from build123d import *

# Parameters (mm, degrees)
SKETCH_1_W          = 145
SKETCH_1_H          = 163.96571483
F_145X120X4MM_DEPTH = 4
SKETCH_2_R          = 2.75
M3_90X70MM_DEPTH    = 162.686711765
FILLET_R5_R         = 5


with BuildPart() as part:
    # 草图1 → 承托板_145x120x4mm (new body)
    with BuildSketch(Plane(origin=(0, 0, 0), x_dir=(1, 0, 0), z_dir=(0, 1, 0))):
        with Locations((0, -62.482857415)):
            Rectangle(SKETCH_1_W, SKETCH_1_H)
    extrude(amount=F_145X120X4MM_DEPTH)

    # 草图2 → 四个M3连接孔_90x70mm (cut, through all)
    with BuildSketch(Plane(origin=(0, 4, 0), x_dir=(1, 0, 0), z_dir=(0, 1, 0))):
        with Locations(Location((-50, -8, 0), (0, 0, 270))):
            Circle(SKETCH_2_R)
        with Locations(Location((-50, -78, 0), (0, 0, 270))):
            Circle(SKETCH_2_R)
        with Locations(Location((50, -8, 0), (0, 0, 270))):
            Circle(SKETCH_2_R)
        with Locations(Location((50, -78, 0), (0, 0, 270))):
            Circle(SKETCH_2_R)
    extrude(amount=-M3_90X70MM_DEPTH, mode=Mode.SUBTRACT)

    # 四角圆角_R5
    fillet_r5_edges = [part.edges().sort_by_distance(p)[0] for p in [
        (-72.5, 2, -19.5),
        (72.5, 2, -19.5),
        (72.5, 2, 144.46571483),
        (-72.5, 2, 144.46571483),
    ]]
    fillet(fillet_r5_edges, radius=FILLET_R5_R)


solid = part.part
Geometry: final body of the model. Coordinates: model frame, mm. Coordinates: 2 decimals unless noted, no trailing zeros. Write each loop counter-clockwise with the first axis right and the second up, starting at its lowest first coordinate (ties: lowest second). Pieces come first, ordered by that corner, then holes. Notation, with made-up numbers: (27.5, 59) - (34.5, 59) arc R22 ccw to (34.5, 78) - close; hole circle Ø4 at (-25, 4). An arc over 180 degrees is marked (long way). Return JSON: item names as keys, results as strings.
Item 1: Pin query (flat end, axial travel): pin 1 Ø5 at (x, z) = (-50, 78) entering from +Y. Return the tip coordinate at first contact, or that it passes through.
Completed:
{"pin 1": "passes through"}
Item 2: Pull-direction query (X, two-part tool) for faces 1 (the face through (-71.074, 2.028, 142.962)), 2 (the face through (-48.141, 2.028, 75.973)), 3 (the face through (-47.273, 2.028, 7.642)), 4 (the face through (-1, 0, 61)); classes: +X half, -X half, draft (parallel to the pull), parting line (faces both ways), or undercut.
Completed:
{"face 1": "-X half", "face 2": "undercut", "face 3": "undercut", "face 4": "draft"}
Item 3: Section query B-B (z = 78). Output: boundary loops of the cut face in (x, y), and give its area (3 significant figures).
Completed:
{"outline": "(-72.5, 0) - (-52.75, 0) - (-52.75, 4) - (-72.5, 4) - close; (-47.25, 0) - (47.25, 0) - (47.25, 4) - (-47.25, 4) - close; (52.75, 0) - (72.5, 0) - (72.5, 4) - (52.75, 4) - close", "area": "536 mm2"}
Item 4: Line query: L1, parallel to X at y = 1.3, z = 78. Output: solid intervals per line, ascending.
Completed:
{"L1": "x = -72.5 to -52.75, -47.25 to 47.25, 52.75 to 72.5"}
Item 5: Section query A-A (x = -50). Output: boundary loops of the cut face in (y, z), and give its area (3 significant figures).
Completed:
{"outline": "(0, -19.5) - (4, -19.5) - (4, 5.25) - (0, 5.25) - close; (0, 10.75) - (4, 10.75) - (4, 75.25) - (0, 75.25) - close; (0, 80.75) - (4, 80.75) - (4, 144.47) - (0, 144.47) - close", "area": "612 mm2"}
